Input: part model. Units: mm. Frame: model coordinates. A direction names the side the tool comes from. Give positions to 0.01 mm unless a question says otherwise; leave off trailing zeros. Loops run counter-clockwise (first coordinate to the right, second up) from the corner with the lowest first, then second, coordinate; pieces in that order, holes last. Notation, with made-up numbers: (60.5, 58) - (116.5, 58) arc R17 cw to (116.5, 83) - close; hole circle Ø4 at (-20.5, -26). An arc over 180 degrees is marked (long way). Answer as a JSON object with one key per item and string values.
from build123d import *
from build123d.topology import SkipClean

# Parameters (mm, degrees)
CROQUIS1_R                = 15
CROQUIS1_R_2              = 7.5
SALIENTE_EXTRUIR1_DEPTH   = 20
SALIENTE_EXTRUIR1_2_DEPTH = 20
SALIENTE_EXTRUIR1_3_DEPTH = 20
CROQUIS1_R_3              = 20
CROQUIS1_R_4              = 4
SALIENTE_EXTRUIR1_4_DEPTH = 20
SALIENTE_EXTRUIR2_DEPTH   = 10
CORTAR_EXTRUIR2_START     = -10
CORTAR_EXTRUIR2_DEPTH     = 10
CORTAR_EXTRUIR3_START     = -10
CROQUIS6_R                = 7.5
CROQUIS6_R_2              = 4
CORTAR_EXTRUIR3_DEPTH     = 10


with BuildPart() as part:
    # Croquis1 → Saliente-Extruir1 (new body)
    with BuildSketch(Plane.XY):
        with Locations((0, -80)):
            Circle(CROQUIS1_R)
        with Locations((0, -80)):
            Circle(CROQUIS1_R_2, mode=Mode.SUBTRACT)
    extrude(amount=SALIENTE_EXTRUIR1_DEPTH)



with BuildPart() as body_2:
    # Croquis1 → Saliente-Extruir1 2 (new body)
    with BuildSketch(Plane.XY):
        with Locations((55, -65)):
            Circle(CROQUIS1_R)
        with Locations((55, -65)):
            Circle(CROQUIS1_R_2, mode=Mode.SUBTRACT)
    extrude(amount=SALIENTE_EXTRUIR1_2_DEPTH)


with BuildPart() as body_3:
    # Croquis1 → Saliente-Extruir1 3 (new body)
    with BuildSketch(Plane.XY):
        with Locations(Location((-55, -65, 0), (0, 0, 180))):
            Circle(CROQUIS1_R)
        with Locations(Location((-55, -65, 0), (0, 0, 180))):
            Circle(CROQUIS1_R_2, mode=Mode.SUBTRACT)
    extrude(amount=SALIENTE_EXTRUIR1_3_DEPTH)


with BuildPart() as body_4:
    # Croquis1 → Saliente-Extruir1 4 (new body)
    with BuildSketch(Plane.XY):
        with BuildLine():
            ThreePointArc((29.967741935, -7.933123174), (39, 0), (29.967741935, 7.933123174))
            ThreePointArc((29.967741935, 7.933123174), (26.846787517, 15.5), (21.854157167, 21.986264223))
            ThreePointArc((21.854157167, 21.986264223), (19.5, 33.774990748), (8.113584768, 29.919387397))
            ThreePointArc((8.113584768, 29.919387397), (0, 31), (-8.113584768, 29.919387397))
            ThreePointArc((-8.113584768, 29.919387397), (-19.5, 33.774990748), (-21.854157167, 21.986264223))
            ThreePointArc((-21.854157167, 21.986264223), (-26.846787517, 15.5), (-29.967741935, 7.933123174))
            ThreePointArc((-29.967741935, 7.933123174), (-39, 0), (-29.967741935, -7.933123174))
            ThreePointArc((-29.967741935, -7.933123174), (-26.846787517, -15.5), (-21.854157167, -21.986264223))
            ThreePointArc((-21.854157167, -21.986264223), (-19.5, -33.774990748), (-8.113584768, -29.919387397))
            ThreePointArc((-8.113584768, -29.919387397), (0, -31), (8.113584768, -29.919387397))
            ThreePointArc((8.113584768, -29.919387397), (19.5, -33.774990748), (21.854157167, -21.986264223))
            ThreePointArc((21.854157167, -21.986264223), (26.846787517, -15.5), (29.967741935, -7.933123174))
        make_face()
        Circle(CROQUIS1_R_3, mode=Mode.SUBTRACT)
        with Locations((31, 0)):
            Circle(CROQUIS1_R_4, mode=Mode.SUBTRACT)
        with Locations((15.5, -26.846787517)):
            Circle(CROQUIS1_R_4, mode=Mode.SUBTRACT)
        with Locations((-15.5, -26.846787517)):
            Circle(CROQUIS1_R_4, mode=Mode.SUBTRACT)
        with Locations((-31, 0)):
            Circle(CROQUIS1_R_4, mode=Mode.SUBTRACT)
        with Locations((-15.5, 26.846787517)):
            Circle(CROQUIS1_R_4, mode=Mode.SUBTRACT)
        with Locations((15.5, 26.846787517)):
            Circle(CROQUIS1_R_4, mode=Mode.SUBTRACT)
    extrude(amount=SALIENTE_EXTRUIR1_4_DEPTH)


with BuildPart() as part_1:
    add(part.part)

    add(body_2.part)  # Saliente-Extruir2 merges body 2

    add(body_3.part)  # Saliente-Extruir2 merges body 3

    add(body_4.part)  # Saliente-Extruir2 merges body 4
    # Croquis2 → Saliente-Extruir2 (add)
    with BuildSketch(Plane.XY):
        with BuildLine():
            Line((39, 0), (52.017194873, -40.678733978))
            ThreePointArc((52.017194873, -40.678733978), (55.61045151, -47.041283696), (61.436740692, -51.451259495))
            ThreePointArc((61.436740692, -51.451259495), (69.632687852, -68.29915841), (55, -80))
            ThreePointArc((55, -80), (0, -95), (-55, -80))
            ThreePointArc((-55, -80), (-69.632687852, -68.29915841), (-61.436740692, -51.451259495))
            ThreePointArc((-61.436740692, -51.451259495), (-55.61045151, -47.041283696), (-52.017194873, -40.678733978))
            Line((-52.017194873, -40.678733978), (-39, 0))
            Line((-39, 0), (39, 0))
        make_face()
    extrude(amount=SALIENTE_EXTRUIR2_DEPTH)

    # Croquis5 → Cortar-Extruir2 (cut)
    with SkipClean():  # the faces are left unmerged after this step: merging them gives an invalid solid
        with BuildSketch(Plane.XY.offset(10).offset(CORTAR_EXTRUIR2_START)):
            with BuildLine():
                Line((-20, 0), (20, 0))
                ThreePointArc((20, 0), (0, -20), (-20, 0))
            make_face()
        extrude(amount=CORTAR_EXTRUIR2_DEPTH, mode=Mode.SUBTRACT)
    add(part_1.part.scale(1), mode=Mode.REPLACE)  # the faces are merged on a copy

    # Croquis6 → Cortar-Extruir3 (cut)
    with SkipClean():  # the faces are left unmerged after this step: merging them gives an invalid solid
        with BuildSketch(Plane.XY.offset(10).offset(CORTAR_EXTRUIR3_START)):
            with Locations(Location((-55, -65, 0), (0, 0, 180))):
                Circle(CROQUIS6_R)
            with Locations((0, -80)):
                Circle(CROQUIS6_R)
            with Locations((55, -65)):
                Circle(CROQUIS6_R)
            with Locations((15.5, -26.846787517)):
                Circle(CROQUIS6_R_2)
            with Locations((-15.5, -26.846787517)):
                Circle(CROQUIS6_R_2)
            with BuildLine():
                Line((-35, 0), (-27, 0))
                ThreePointArc((-27, 0), (-31, -4), (-35, 0))
            make_face()
            with BuildLine():
                Line((27, 0), (35, 0))
                ThreePointArc((35, 0), (31, -4), (27, 0))
            make_face()
        extrude(amount=CORTAR_EXTRUIR3_DEPTH, mode=Mode.SUBTRACT)
    add(part_1.part.scale(1), mode=Mode.REPLACE)  # the faces are merged on a copy


solid = part_1.part
Item 1: Contact query for flat-ended pins moving along their axis: P1, Ø1, axis at y = 3, z = 7, coming from the +X side; P2, Ø12, axis at y = -42.5, z = 5, coming from the +X side; P3, Ø4, axis at x = 22.5, z = 13.5, coming from the +Y side. Output: stop coordinate, or through.
Geometry check:
{"P1": "stops at x = 38.6", "P2": "stops at x = 57.04", "P3": "stops at y = 33.09"}
Item 2: Material intervals for line 1 (X direction, y = -26.5, z = 11); line 2 (X direction, y = 0, z = 12); line 3 (Y direction, x = 55, z = 16.25), sorted ascending. Write a range as [from, to].
Geometry check:
{"line 1": "x = [-23.49, -19.48], [-11.52, 11.52], [19.48, 23.49]", "line 2": "x = [-39, -35], [-27, -20], [20, 27], [35, 39]", "line 3": "y = [-80, -72.5], [-57.5, -50]"}
Item 3: Access query for faces 5 (the face through (0, -31, 15)), 6 (the face through (1, -44, 0)). Directions: +Z, -Z, +X, -X, +Y, -Y. A direction counts if a zero-diameter tool reaches every point of the face in a straight line with its end or side. Return the directions, or none.
Geometry check:
{"face 5": "+Z", "face 6": "-Z, +X, -X, +Y, -Y"}
Item 4: Cut plane C-C (y = 24.5). Return loops of the section in (x, z).
Geometry check:
{"outline": "(-23.15, 0) - (-18.74, 0) - (-18.74, 20) - (-23.15, 20) - close; (-12.26, 0) - (12.26, 0) - (12.26, 20) - (-12.26, 20) - close; (18.74, 0) - (23.15, 0) - (23.15, 20) - (18.74, 20) - close"}
Item 5: Mould query, pull axis Y, two halves, no side actions, for faces 1 (the face through (19.33, -33.87, 14.93)), 2 (the face through (-38.363, 3.127, 12.082)), 3 (the face through (0.808, -94.997, 4.93)), 4 (the face through (-4.336, -19.524, 9.86)). Classes: released by +Y, released by -Y, zero draft, split by the parting line, or undercut.
Geometry check:
{"face 1": "undercut", "face 2": "split by the parting line", "face 3": "released by -Y", "face 4": "undercut"}
Item 6: Cut plane A-A (z = 17.75). Give the number of separate pieces and of enclosed holes in the cut face, then the cut area to 3 significant figures.
Geometry check:
{"separate pieces": "4", "enclosed holes": "10", "area": "3,690 mm2"}
Item 7: Cut plane D-D (y = -44). Return loops of the section in (x, z), then the cut area to 3 significant figures.
Geometry check:
{"outline": "(-53.46, 0) - (53.46, 0) - (53.46, 10) - (-53.46, 10) - close", "area": "1,070 mm2"}
